Job drawing, mm, ordinate dimensions from the low corner. One solid piece. A direction names the side the tool comes from. Round coordinates to 2 decimals unless told otherwise and drop trailing zeros. Write each loop counter-clockwise with the first axis right and the second up, starting at its lowest first coordinate (ties: lowest second). Pieces come first, ordered by that corner, then holes. Notation, with made-up numbers: M 78.5,55.25 L 134.5,55.25 A15 ccw 134.5,62.25 Z; hole C 58.25,-2.5 d10. An arc over 180 degrees is marked long. One line per item, written item: value. Start each with the question number.
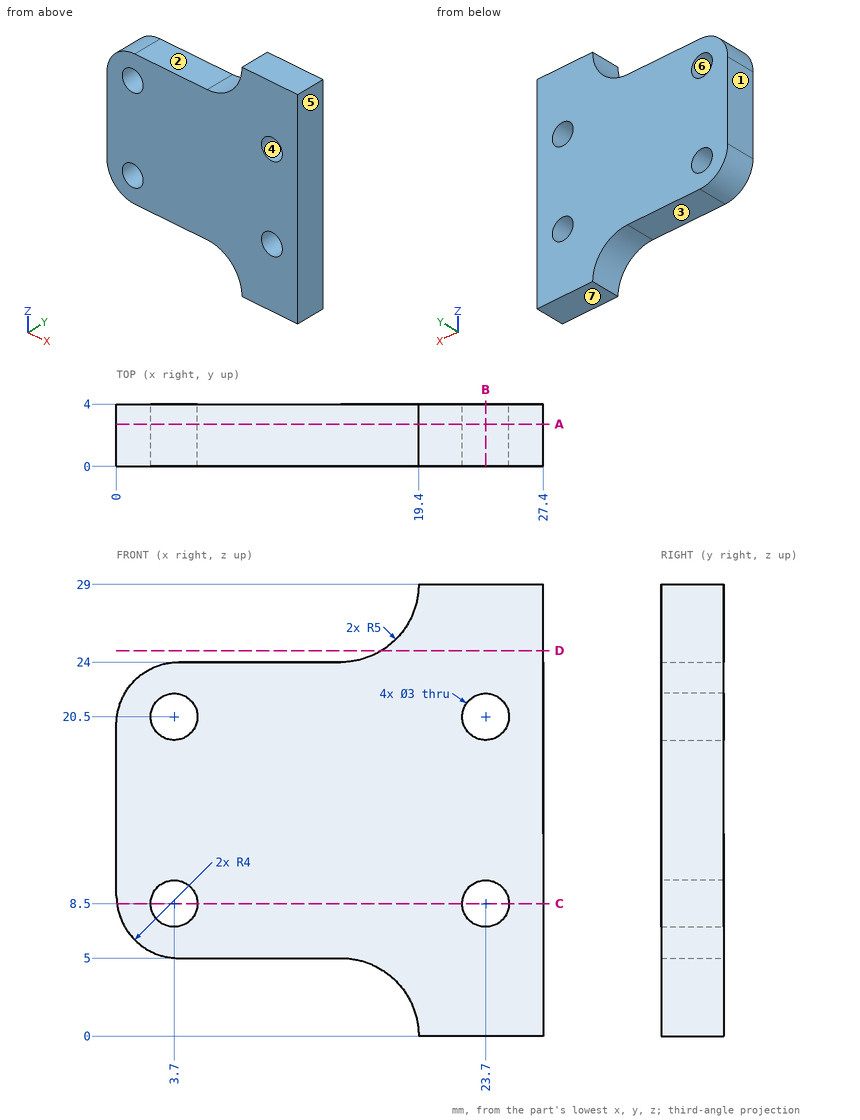
Item 1: Which spindle directions (+Z, -Z, +X, -X, +Y, -Y) get a long thin tool onto all of the face, cutting with end or side? Do the marked faces 1, 2 and 3. Say none if no direction does.
Item 2: Drop flat-ended pins along their axis: pin 1 (1.8 mm diameter, centred on x = 3.7, z = 20.5, fed in from -Y); pin 2 (1.2 mm diameter, centred on x = 9.5, y = 2.5, fed in from +Z). Give the stop position or say it passes through.
Item 3: Drill centre lines: line 1 (X direction, y = 2.05, z = 20.5); line 2 (Z direction, x = 3.5, y = 0.6); line 3 (Z direction, x = 24.75, y = 1.6). Where is each one in solid material? Low to high.
Item 4: Cut at D-D, the plane z = 24.75. Write the cut outline in (x, y), plus the area to 3 significant figures.
Item 5: Cut at C-C, the plane z = 8.5. Write the cut outline in (x, y), plus the area to 3 significant figures.
Item 6: Cut at B-B, the plane x = 23.7. Write the cut outline in (y, z), plus the area to 3 significant figures.
Item 7: Two-plate mould, pull along Z, no slides. Class the marked faces 4, 5, 6 and 7: pulls with the +Z half, pulls with the -Z half, needs draft (parallel to the pull), parting line crosses it, or undercut.
Item 8: Cut at A-A, the plane y = 2.7. Count the separate pieces of the cut face and the enclosed holes in it, plus the area to 3 significant figures.
Computed values:
1. face 1: +Z, -Z, -X, +Y, -Y
1. face 2: +Z, -X, +Y, -Y
1. face 3: -Z, -X, +Y, -Y
2. pin 1: passes through
2. pin 2: stops at z = 24
3. line 1: x = 0.03 to 2.2, 5.2 to 22.2, 25.2 to 27.4
3. line 2: z = 5.03 to 7.01, 9.99 to 19.01, 21.99 to 23.97
3. line 3: z = 0 to 7.43, 9.57 to 19.43, 21.57 to 29
4. outline: M 17.03,0 L 27.4,0 L 27.4,4 L 17.03,4 Z
4. area: 41.5 mm2
5. outline: M 0.03,0 L 2.2,0 L 2.2,4 L 0.03,4 Z; M 5.2,0 L 22.2,0 L 22.2,4 L 5.2,4 Z; M 25.2,0 L 27.4,0 L 27.4,4 L 25.2,4 Z
5. area: 85.5 mm2
6. outline: M 0,0 L 4,0 L 4,7 L 0,7 Z; M 0,10 L 4,10 L 4,19 L 0,19 Z; M 0,22 L 4,22 L 4,29 L 0,29 Z
6. area: 92.0 mm2
7. face 4: undercut
7. face 5: needs draft
7. face 6: undercut
7. face 7: pulls with the -Z half
8. separate pieces: 1
8. enclosed holes: 4
8. area: 576 mm2
